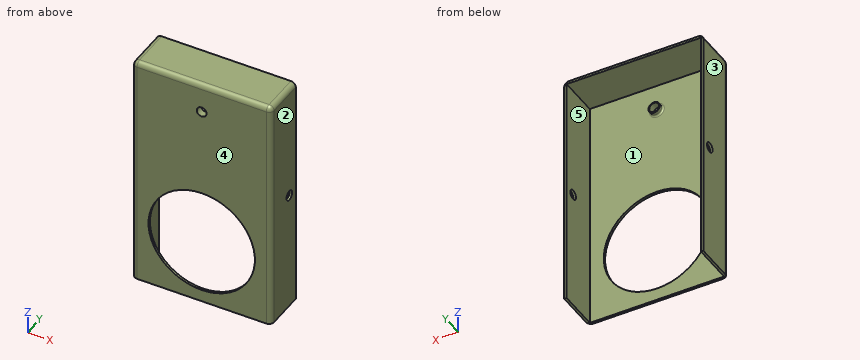
from build123d import *

# Parameters (mm, degrees)
SKETCH1_W               = 85
SKETCH1_H               = 145
SKETCH1_R               = 32.5
SKETCH1_R_2             = 3
BOSS_EXTRUDE1_DEPTH     = 1.5
SKETCH2_W               = 82
SKETCH2_H               = 1.5
BOSS_EXTRUDE2_DEPTH     = 25
CUT_EXTRUDE1_DEPTH      = 89.117818856
CUT_EXTRUDE1_DEPTH_BACK = 89.117818856
SKETCH3_R               = 3
FILLET1_R               = 3
SKETCH4_R               = 3.5
SKETCH4_R_2             = 3
BOSS_EXTRUDE3_DEPTH     = 3
FILLET2_R               = 1


with BuildPart() as part:
    # Sketch1 → Boss-Extrude1 (new body)
    with BuildSketch(Plane(origin=(0, 0, 0), x_dir=(1, 0, 0), z_dir=(0, 1, 0))):
        Rectangle(SKETCH1_W, SKETCH1_H)
        with Locations(Location((0, 32.5, 0), (0, 0, 270))):
            Circle(SKETCH1_R, mode=Mode.SUBTRACT)
        with Locations(Location((0, -54.5, 0), (0, 0, 270))):
            Circle(SKETCH1_R_2, mode=Mode.SUBTRACT)
    extrude(amount=BOSS_EXTRUDE1_DEPTH)

    # Sketch2 → Boss-Extrude2 (add)
    with BuildSketch(Plane(origin=(0, 1.5, 0), x_dir=(1, 0, 0), z_dir=(0, 1, 0))):
        Polygon((-42.5, 72.5), (-42.5, -72.5), (-41, -72.5), (-41, -71), (-41, 72.5), align=None)
        with Locations((0, -71.75)):
            Rectangle(SKETCH2_W, SKETCH2_H)
        Polygon((41, -71), (41, -72.5), (42.5, -72.5), (42.5, 72.5), (41, 72.5), align=None)
    extrude(amount=BOSS_EXTRUDE2_DEPTH)

    # Sketch3 → Cut-Extrude1 (cut, two sides: drawn at the far end of the back side and taken through both)
    with BuildSketch(Plane(origin=(0, 0, 0), x_dir=(0, 0, -1), z_dir=(1, 0, 0)).offset(-CUT_EXTRUDE1_DEPTH_BACK)):
        with Locations((-1.5, 19.5)):
            Circle(SKETCH3_R)
    extrude(amount=CUT_EXTRUDE1_DEPTH + CUT_EXTRUDE1_DEPTH_BACK, mode=Mode.SUBTRACT)

    # Fillet1
    fillet1_edges = [part.edges().sort_by_distance(p)[0] for p in [
        (42.5, 0, 0),
        (0, 0, 72.5),
        (-42.5, 0, 0),
        (42.5, 13.25, 72.5),
        (-42.5, 13.25, 72.5),
    ]]
    fillet(fillet1_edges, radius=FILLET1_R)

    # Sketch4 → Boss-Extrude3 (add)
    with BuildSketch(Plane(origin=(0, 1.5, 0), x_dir=(1, 0, 0), z_dir=(0, 1, 0))):
        with Locations(Location((0, -54.5, 0), (0, 0, 270))):
            Circle(SKETCH4_R)
        with Locations(Location((0, -54.5, 0), (0, 0, 270))):
            Circle(SKETCH4_R_2, mode=Mode.SUBTRACT)
    extrude(amount=BOSS_EXTRUDE3_DEPTH)

    # Fillet2
    fillet2_edges = [part.edges().sort_by_distance(p)[0] for p in [
        (0, 1.5, 51),
    ]]
    fillet(fillet2_edges, radius=FILLET2_R)


solid = part.part
Here's how the part is built. I have some questions about the finished solid (model axes, mm). Face numbers are marked on the shaded views. A direction names the side the tool comes from. Round coordinates to 2 decimals unless told otherwise and drop trailing zeros. Write each loop counter-clockwise with the first axis right and the second up, starting at its lowest first coordinate (ties: lowest second). Pieces come first, ordered by that corner, then holes.
1. Suppose I cut it at C-C (x = 0). List the corners of the cut face in (y, z) for me.
2. For the marked faces 4 and 5, which set-ups out of +Z, -Z, +X, -X, +Y, -Y let a thin tool reach every point of the face, with its end or its side?
3. If we mould it in two halves opening along X, with no side actions, what happens to the marked faces 1, 2 and 3? For each: released by +X, released by -X, zero draft, split by the parting line, or undercut.
4. Suppose I cut it at D-D (z = 1.5). List the corners of the cut face in (x, y) for me, and give its area (3 significant figures).
5. Will this pin go through, and if not, where does the flat tip stop? pin 1 Ø4 at (x, z) = (24, 1.5) entering from +Y.
6. Suppose I cut it at B-B (x = -30). List the corners of the cut face in (y, z) for me.
7. I need wall thicknesses on L1, parallel to X at y = 8, z = -7; L2, parallel to X at y = 2.45, z = 54.5; L3, parallel to Y at x = 16, z = 34. Which ranges of each line are inside material? Lowest first, please.
8. Suppose I cut it at A-A (z = -32.5). List the corners of the cut face in (x, y) for me, and give its area (3 significant figures).
Answer sheet:
1. outline: (0, -72.5) - (1.5, -72.5) - (1.5, -65) - (0, -65) - close; (0, 0) - (1.5, 0) - (1.5, 50) arc R1 cw to (2.5, 51) - (4.5, 51) - (4.5, 51.5) - (0, 51.5) - close; (0, 57.5) - (4.5, 57.5) - (4.5, 58) - (2.5, 58) arc R1 cw to (1.5, 59) - (1.5, 71) - (26.5, 71) - (26.5, 72.5) - (3, 72.5) arc R3 ccw to (0, 69.5) - close
2. face 4: +Z, -Z, +X, -X, -Y
2. face 5: -Z, +Y
3. face 1: undercut
3. face 2: released by +X
3. face 3: released by -X
4. outline: (-42.5, 3) arc R3 ccw to (-39.5, 0) - (39.5, 0) arc R3 ccw to (42.5, 3) - (42.5, 16.5) - (41, 16.5) - (41, 1.5) - (-41, 1.5) - (-41, 16.5) - (-42.5, 16.5) - close; (-42.5, 22.5) - (-41, 22.5) - (-41, 26.5) - (-42.5, 26.5) - close; (41, 22.5) - (42.5, 22.5) - (42.5, 26.5) - (41, 26.5) - close
4. area: 181 mm2
5. pin 1: stops at y = 1.5
6. outline: (0, -72.5) - (1.5, -72.5) - (1.5, -45) - (0, -45) - close; (0, -20) - (1.5, -20) - (1.5, 71) - (26.5, 71) - (26.5, 72.5) - (3, 72.5) arc R3 ccw to (0, 69.5) - close
7. L1: x = -42.5 to -41, 41 to 42.5
7. L2: x = -42.45 to -41, -3.5 to -3, 3 to 3.5, 41 to 42.45
7. L3: y = 0 to 1.5
8. outline: (-42.5, 3) arc R3 ccw to (-39.5, 0) - (-32.5, 0) - (-32.5, 1.5) - (-41, 1.5) - (-41, 26.5) - (-42.5, 26.5) - close; (32.5, 0) - (39.5, 0) arc R3 ccw to (42.5, 3) - (42.5, 26.5) - (41, 26.5) - (41, 1.5) - (32.5, 1.5) - close
8. area: 101 mm2
